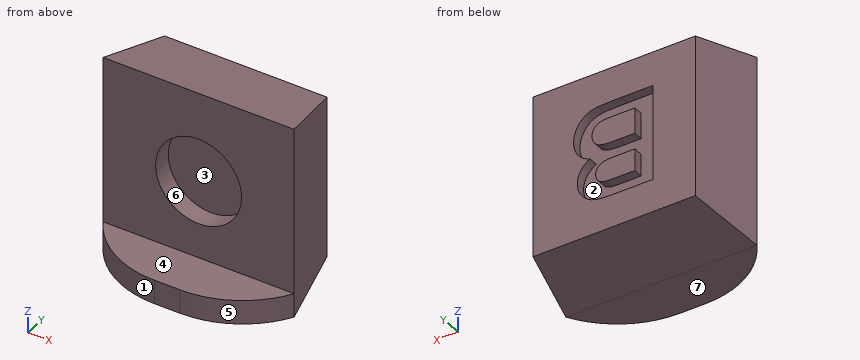
```python
from build123d import *

# Parameters (mm, degrees)
SKETCH1_W               = 8
SKETCH1_H               = 8
BOSS_EXTRUDE1_DEPTH     = 3
CUT_EXTRUDE1_DEPTH      = 12.704699911
CUT_EXTRUDE1_DEPTH_BACK = 12.704699911
CUT_EXTRUDE2_DEPTH      = 11
SKETCH4_R               = 1.8
CUT_EXTRUDE3_DEPTH      = 0.8
SKETCH5_W               = 8
SKETCH5_H               = 1
BOSS_EXTRUDE2_DEPTH     = 2
FILLET1_R               = 4
CUT_EXTRUDE4_DEPTH      = 0.4


with BuildPart() as part:
    # Sketch1 → Boss-Extrude1 (new body)
    with BuildSketch(Plane(origin=(0, 0, 0), x_dir=(1, 0, 0), z_dir=(0, 1, 0))):
        with Locations((4, 4)):
            Rectangle(SKETCH1_W, SKETCH1_H)
    extrude(amount=BOSS_EXTRUDE1_DEPTH)

    # Sketch2 → Cut-Extrude1 (cut, two sides: drawn at the far end of the back side and taken through both)
    with BuildSketch(Plane.XY.offset(-CUT_EXTRUDE1_DEPTH_BACK)):
        Polygon((0, 0), (0.6, 3), (0, 3), align=None)
        Polygon((8, 0), (7.4, 3), (8, 3), align=None)
    extrude(amount=CUT_EXTRUDE1_DEPTH + CUT_EXTRUDE1_DEPTH_BACK, mode=Mode.SUBTRACT)

    # Sketch3 → Cut-Extrude2 (cut)
    with BuildSketch(Plane(origin=(0, 0, 0), x_dir=(0, 0, -1), z_dir=(1, 0, 0))):
        Polygon((0, 0), (0.6, 3), (0, 3), align=None)
        Polygon((8, 3), (7.4, 3), (8, 0), align=None)
    extrude(amount=CUT_EXTRUDE2_DEPTH, mode=Mode.SUBTRACT)

    # Sketch4 → Cut-Extrude3 (cut)
    with BuildSketch(Plane.XZ):
        with Locations(Location((4, -3.75, 0), (0, 0, 270))):
            Circle(SKETCH4_R)
    extrude(amount=-CUT_EXTRUDE3_DEPTH, mode=Mode.SUBTRACT)

    # Sketch5 → Boss-Extrude2 (add)
    with BuildSketch(Plane.XZ):
        with Locations((4, -7.5)):
            Rectangle(SKETCH5_W, SKETCH5_H)
    extrude(amount=BOSS_EXTRUDE2_DEPTH)

    # Fillet1
    # the kernel refuses this fillet: 4 mm, written as the material it takes off along each edge
    with BuildSketch(Plane(origin=(8, -2, -16.660254038), x_dir=(0, 1, 0), z_dir=(0, 0, 1)), Plane(origin=(0, -2, 1.660254038), x_dir=(0, 1, 0), z_dir=(0, 0, -1))) as fillet1_piece_1:
        with BuildLine():
            CenterArc((4, 3.464101615), FILLET1_R, 180, 60)
            Line((0, 3.464101615), (-0.08, 3.464101615))
            Line((-0.08, 3.464101615), (-0.08, 0))
            Line((-0.08, 0), (0, -0.08))
            ThreePointArc((0, -0.08), (1, -0.08), (1.96, -0.069282032))
            Line((1.96, -0.069282032), (2, 0))
        make_face()
    extrude(amount=18.320508076, mode=Mode.SUBTRACT)

    # Sketch6 → Cut-Extrude4 (cut)
    with BuildSketch(Plane(origin=(0, 3, 0), x_dir=(1, 0, 0), z_dir=(0, 1, 0))):
        with BuildLine():
            Line((2.366875023, 6.025988971), (3.978253228, 6.025988971))
            add(Edge.make_bspline(
                [(3.978253228, 6.025988971), (4.016981522, 6.025758539), (4.091770291, 6.025313549), (4.200234262, 6.02407341), (4.300910244, 6.020431423), (4.393955008, 6.01730407), (4.479059098, 6.009990491), (4.556891378, 6.004244483), (4.627206795, 5.996339471), (4.710040188, 5.983546816), (4.806360793, 5.963648743), (4.915152558, 5.926842691), (5.018276483, 5.880857129), (5.114182519, 5.822393524), (5.203189243, 5.754016663), (5.28597738, 5.676271174), (5.358728101, 5.58601543), (5.424238976, 5.487508268), (5.479534837, 5.380666952), (5.517612886, 5.26572697), (5.541913225, 5.144795761), (5.544858568, 5.061898711), (5.546362202, 5.019578715)],
                knots=[0, 0, 0, 0, 1.096610875, 2.117681168, 3.071055591, 3.949137991, 4.753059115, 5.489127199, 6.15892391, 6.75575099, 7.862330316, 8.938514814, 10.001276227, 11.05313779, 12.110449801, 13.174958802, 14.260456508, 15.384725817, 16.521138801, 17.654729897, 18.802709851, 20, 20, 20, 20], degree=3))
            add(Edge.make_bspline(
                [(5.546362202, 5.019578715), (5.544802721, 4.973493311), (5.541727769, 4.882623117), (5.513106772, 4.749371009), (5.467516851, 4.621879661), (5.40315043, 4.502217288), (5.324314646, 4.392405777), (5.231065087, 4.295977947), (5.12477188, 4.213520097), (5.044958184, 4.17248881), (5.004695536, 4.151790253)],
                knots=[0, 0, 0, 0, 1.023065178, 2.01725758, 3.014298905, 4.023406433, 5.026736079, 6.009055718, 6.99565244, 8, 8, 8, 8], degree=3))
            add(Edge.make_bspline(
                [(5.004695536, 4.151790253), (5.0318132, 4.142553707), (5.085431798, 4.12429068), (5.162178571, 4.090754541), (5.234086142, 4.051862796), (5.301118401, 4.008841827), (5.363784101, 3.961377137), (5.420252395, 3.907894911), (5.473763466, 3.851437899), (5.520742036, 3.789172127), (5.563264851, 3.724075672), (5.599360366, 3.65512964), (5.630616076, 3.583992364), (5.656755805, 3.509943884), (5.675388869, 3.432487562), (5.69031884, 3.352599145), (5.697956597, 3.269724954), (5.699451608, 3.213768347), (5.700208356, 3.185444099)],
                knots=[0, 0, 0, 0, 1.072651974, 2.1209089, 3.132484228, 4.131466326, 5.101889999, 6.071643115, 7.041396231, 8.011819904, 8.988565287, 9.95070344, 10.922775742, 11.897213062, 12.887138018, 13.903598663, 14.938838629, 16, 16, 16, 16], degree=3))
            add(Edge.make_bspline(
                [(5.700208356, 3.185444099), (5.698598844, 3.140212221), (5.695387249, 3.049957264), (5.671387404, 2.915316113), (5.630853991, 2.783046233), (5.575963383, 2.654005704), (5.507783193, 2.532330941), (5.427626978, 2.4212421), (5.334105775, 2.324584109), (5.230539132, 2.239414342), (5.113835126, 2.16890592), (4.984093466, 2.114745557), (4.842134035, 2.073828468), (4.742124288, 2.060236169), (4.690592972, 2.053232561)],
                knots=[0, 0, 0, 0, 0.975059807, 1.945618526, 2.93861228, 3.952760547, 4.963632603, 5.940527786, 6.897802811, 7.855787948, 8.824773195, 9.82606706, 10.879852914, 12, 12, 12, 12], degree=3))
            add(Edge.make_bspline(
                [(4.690592972, 2.053232561), (4.670833027, 2.051565703), (4.625472552, 2.047739302), (4.548543711, 2.042982046), (4.453955886, 2.039386091), (4.341791209, 2.035134329), (4.211704387, 2.032064432), (4.063991072, 2.029968108), (3.898399223, 2.027247493), (3.782207382, 2.026423), (3.72104169, 2.025988971)],
                knots=[0, 0, 0, 0, 0.490565993, 1.126131979, 1.906526787, 2.832178623, 3.902933831, 5.125497984, 6.486805064, 8, 8, 8, 8], degree=3))
            Line((3.72104169, 2.025988971), (2.366875023, 2.025988971))
            Line((2.366875023, 2.025988971), (2.366875023, 6.025988971))
        make_face()
        with BuildLine():
            Line((3.136105792, 5.359322304), (3.136105792, 4.436245381))
            Line((3.136105792, 4.436245381), (3.692996818, 4.436245381))
            add(Edge.make_bspline(
                [(3.692996818, 4.436245381), (3.732259986, 4.43615888), (3.807047978, 4.435994114), (3.91334909, 4.43709824), (4.008173732, 4.437613694), (4.091249283, 4.439126475), (4.162558686, 4.441623123), (4.221845003, 4.444116229), (4.269450826, 4.446003799), (4.297170592, 4.448699163), (4.309182715, 4.449867176)],
                knots=[0, 0, 0, 0, 1.528479216, 2.911428072, 4.138414629, 5.21998762, 6.145918986, 6.915989543, 7.530253335, 8, 8, 8, 8], degree=3))
            add(Edge.make_bspline(
                [(4.309182715, 4.449867176), (4.3438238, 4.455079871), (4.41040184, 4.465098351), (4.503567155, 4.494454854), (4.584375726, 4.536913614), (4.653724553, 4.58976356), (4.708773054, 4.654604252), (4.749170144, 4.72919452), (4.772805412, 4.813847791), (4.775653451, 4.873327339), (4.777131433, 4.904194099)],
                knots=[0, 0, 0, 0, 1.162079002, 2.233444551, 3.225172046, 4.179556897, 5.110707885, 6.027301426, 6.976273101, 8, 8, 8, 8], degree=3))
            add(Edge.make_bspline(
                [(4.777131433, 4.904194099), (4.776203651, 4.934000177), (4.774422539, 4.991220438), (4.752297006, 5.072236392), (4.719032932, 5.144995211), (4.670409719, 5.207709385), (4.609395094, 5.260672186), (4.534716376, 5.302043411), (4.446732173, 5.330510733), (4.38335661, 5.340467498), (4.3500481, 5.345700509)],
                knots=[0, 0, 0, 0, 1.044241546, 2.004684189, 2.928111627, 3.838334562, 4.769594837, 5.748424953, 6.81663206, 8, 8, 8, 8], degree=3))
            add(Edge.make_bspline(
                [(4.3500481, 5.345700509), (4.336967148, 5.34687206), (4.306041436, 5.349641817), (4.252292165, 5.35144236), (4.183926257, 5.353976507), (4.100595234, 5.356449705), (4.002296842, 5.357959731), (3.889310645, 5.358468661), (3.761641688, 5.359577608), (3.671629596, 5.359410545), (3.624086561, 5.359322304)],
                knots=[0, 0, 0, 0, 0.433943041, 1.02591908, 1.776648879, 2.694999143, 3.780816848, 5.02540149, 6.428861738, 8, 8, 8, 8], degree=3))
            Line((3.624086561, 5.359322304), (3.136105792, 5.359322304))
        make_face(mode=Mode.SUBTRACT)
        with BuildLine():
            Line((3.136105792, 3.769578715), (3.136105792, 2.692655638))
            Line((3.136105792, 2.692655638), (3.921362202, 2.692655638))
            add(Edge.make_bspline(
                [(3.921362202, 2.692655638), (3.957955896, 2.692474114), (4.027408125, 2.692129595), (4.126486109, 2.694437139), (4.214933064, 2.69519802), (4.293162962, 2.698994102), (4.360764719, 2.701865798), (4.418016495, 2.705445849), (4.464471269, 2.711139165), (4.491885355, 2.715559172), (4.503894254, 2.717495381)],
                knots=[0, 0, 0, 0, 1.504773752, 2.85595359, 4.075347731, 5.141676974, 6.076328919, 6.858106537, 7.499786952, 8, 8, 8, 8], degree=3))
            add(Edge.make_bspline(
                [(4.503894254, 2.717495381), (4.534390702, 2.723929926), (4.593642924, 2.736431746), (4.675765739, 2.772305806), (4.749780788, 2.817800627), (4.813883543, 2.876271003), (4.866572685, 2.946316906), (4.904617992, 3.02809262), (4.927561873, 3.120636015), (4.929805566, 3.185839411), (4.930977587, 3.219899227)],
                knots=[0, 0, 0, 0, 1.031056579, 2.003262591, 2.954260215, 3.900917722, 4.862741126, 5.841340256, 6.872396835, 8, 8, 8, 8], degree=3))
            add(Edge.make_bspline(
                [(4.930977587, 3.219899227), (4.930031736, 3.249108452), (4.928190747, 3.305960799), (4.910169932, 3.38739087), (4.88101832, 3.461844609), (4.840421058, 3.528813936), (4.789699747, 3.589139928), (4.726998003, 3.639624345), (4.654607383, 3.681685756), (4.585597801, 3.709395341), (4.520158829, 3.72717269), (4.457743787, 3.73883498), (4.382520906, 3.748066566), (4.294854864, 3.755875466), (4.194389919, 3.762120128), (4.081396073, 3.767043008), (3.95555801, 3.769103428), (3.867409493, 3.769415255), (3.821201946, 3.769578715)],
                knots=[0, 0, 0, 0, 0.992165387, 1.931134082, 2.820086661, 3.700270762, 4.583075858, 5.486803518, 6.423132184, 7.421722103, 8.005700193, 8.727213115, 9.57900282, 10.582332745, 11.720121093, 13.002085041, 14.428489784, 16, 16, 16, 16], degree=3))
            Line((3.821201946, 3.769578715), (3.136105792, 3.769578715))
        make_face(mode=Mode.SUBTRACT)
    extrude(amount=-CUT_EXTRUDE4_DEPTH, mode=Mode.SUBTRACT)


solid = part.part
```
Could you check a few things on this model? Use its own coordinates, in mm. Face numbers are marked on the shaded views. A direction names the side the tool comes from. Coordinates: 2 decimals unless noted, no trailing zeros. Loops run counter-clockwise (first coordinate to the right, second up) from the corner with the lowest first, then second, coordinate; pieces in that order, holes last. Notation, with made-up numbers: M 23.25,16.25 L 43.25,16.25 A14 ccw 43.25,37.25 Z; hole C 33,78 d4. An arc over 180 degrees is marked long. Put each result on its own line as item: value. Start each with the question number.
(1) Will these pins go through, and if not, where does the flat tip stop? P1, Ø1, axis at x = 6, y = 2.5, coming from the +Z side; P2, Ø1.5, axis at y = -0.5, z = -7, coming from the -X side; P3, Ø2, axis at x = 2, z = -3.5, coming from the -Y side; P4, Ø1.5, axis at x = 2, y = 2, coming from the -Z side.
(2) Suppose I cut it at B-B on z = -0.75. Please give me the cut outline in (x, y).
(3) Thinking about a two-plate mould opening in X: for the marked faces 5, 6 and 7, which applies, pulls with the +X half, pulls with the -X half, needs draft (parallel to the pull), parting line crosses it, or undercut?
(4) I need wall thicknesses on line 1 (Y direction, x = 1, z = -2.5); line 2 (X direction, y = 0.45, z = -3.75); line 3 (Y direction, x = 5, z = -4.5). Which ranges of each line are inside material? Lowest first, please. Write a range as from..to.
(5) For the marked faces 1, 2, 3 and 4, which set-ups out of +Z, -Z, +X, -X, +Y, -Y let a thin tool reach every point of the face, with its end or its side?
(6) Suppose I cut it at A-A on y = 0.25. Please give me the cut outline in (x, z).
Solutions:
1. P1: stops at z = -0.4
1. P2: stops at x = 0
1. P3: stops at y = 0
1. P4: stops at z = -7.75
2. outline: M 0,0 L 8,0 L 7.4,3 L 0.6,3 Z
3. face 5: pulls with the +X half
3. face 6: undercut
3. face 7: needs draft
4. line 1: y = 0..3
4. line 2: x = 0.09..2.2, 5.8..7.91
4. line 3: y = 0.8..2.6
5. face 1: +Z, -Z, -X, -Y
5. face 2: +Y
5. face 3: -Y
5. face 4: +Z, +X, -X, -Y
6. outline: M 0.05,-7.95 L 7.95,-7.95 L 7.95,-0.05 L 0.05,-0.05 Z; hole C 4,-3.75 d3.6
